```python
from build123d import *

# Parameters (mm, degrees)
SKETCH1_R           = 4
BOSS_EXTRUDE1_DEPTH = 25
SKETCH2_R           = 10
CUT_EXTRUDE1_DEPTH  = 15


with BuildPart() as part:
    # Sketch1 → Boss-Extrude1 (new body)
    with BuildSketch(Plane(origin=(0, 0, 0), x_dir=(1, 0, 0), z_dir=(0, 1, 0))):
        Polygon((-35, -10), (-30, -10), (-30, -25), (30, -25), (30, -10), (35, -10), (35, 10), (-35, 10), align=None)
        with Locations(Location((-25, 0, 0), (0, 0, 270))):
            Circle(SKETCH1_R, mode=Mode.SUBTRACT)
        with Locations(Location((25, 0, 0), (0, 0, 90))):
            Circle(SKETCH1_R, mode=Mode.SUBTRACT)
    extrude(amount=BOSS_EXTRUDE1_DEPTH)

    # Sketch2 → Cut-Extrude1 (cut)
    with BuildSketch(Plane.XY.offset(25)):
        with Locations((-12.5, 12.5)):
            Circle(SKETCH2_R)
        with Locations(Location((12.5, 12.5, 0), (0, 0, 180))):
            Circle(SKETCH2_R)
    extrude(amount=-CUT_EXTRUDE1_DEPTH, mode=Mode.SUBTRACT)


solid = part.part
```
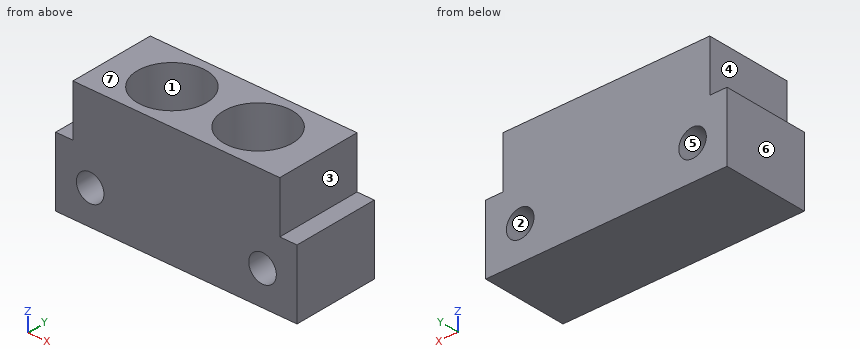
Source: CAD feature listing. Evaluate the final solid. Frame: model axes, mm. Face numbers are marked on the shaded views. A direction names the side the tool comes from. Round coordinates to 2 decimals unless told otherwise and drop trailing zeros. Loops run counter-clockwise (first coordinate to the right, second up) from the corner with the lowest first, then second, coordinate; pieces in that order, holes last. Notation, with made-up numbers: M 88.25,-24 L 135.25,-24 A8 cw 135.25,-18 Z; hole C 75,83.25 d6. An arc over 180 degrees is marked long. Put each result on its own line as item: value.
(1) Access query for the marked faces 1, 2, 3 and 4. Directions: +Z, -Z, +X, -X, +Y, -Y. A direction counts if a zero-diameter tool reaches every point of the face in a straight line with its end or side. Return the directions, or none.
Solutions:
face 1: +Z
face 2: +Y, -Y
face 3: +Z, +X, +Y, -Y
face 4: +Z, -X, +Y, -Y
(2) Ray query, line 1 (X direction, y = 16, z = 0); line 2 (X direction, y = 21, z = 18.5); line 3 (Y direction, x = 12.5, z = 15.25). Return the intervals inside material, ascending. Write a range as [from, to].
Solutions:
line 1: [-35, -29], [-21, 21], [29, 35]
line 2: [-30, -17.77], [-7.23, 7.23], [17.77, 30]
line 3: [0, 2.5], [22.5, 25]
(3) First-contact query: pin 1 (7.5 mm diameter, centred on y = 7.5, z = 18, fed in from +X); pin 2 (3 mm diameter, centred on x = -12, y = 5, fed in from +Z); pin 3 (7.5 mm diameter, centred on y = 9, z = 21, fed in from -X). Flat tips, straight axial feed; report the tip coordinate or a pass-through.
Solutions:
pin 1: x = 30
pin 2: z = 10
pin 3: x = -30
(4) Section C-C, the plane x = 12.5. Return loops of the section in (y, z), and give its area (3 significant figures).
Solutions:
outline: M 0,-10 L 25,-10 L 25,25 L 22.5,25 L 22.5,10 L 2.5,10 L 2.5,25 L 0,25 Z
area: 575 mm²
(5) Section A-A, the plane z = 0. Return loops of the section in (x, y), and give its area (3 significant figures).
Solutions:
outline: M -35,0 L -29,0 L -29,25 L -35,25 Z; M -21,0 L 21,0 L 21,25 L -21,25 Z; M 29,0 L 35,0 L 35,25 L 29,25 Z
area: 1,350 mm²
(6) Section D-D, the plane y = 11.25. Return loops of the section in (x, z).
Solutions:
outline: M -35,-10 L 35,-10 L 35,10 L 30,10 L 30,25 L 22.42,25 L 22.42,10 L 2.58,10 L 2.58,25 L -2.58,25 L -2.58,10 L -22.42,10 L -22.42,25 L -30,25 L -30,10 L -35,10 Z; hole C -25,0 d8; hole C 25,0 d8
(7) Pull-direction query (X, two-part tool) for the marked faces 5, 6 and 7; classes: released by +X, released by -X, zero draft, split by the parting line, or undercut.
Solutions:
face 5: undercut
face 6: released by -X
face 7: zero draft
(8) Section B-B, the plane x = 25. Return loops of the section in (y, z), and give its area (3 significant figures).
Solutions:
outline: M 0,-10 L 25,-10 L 25,-4 L 0,-4 Z; M 0,4 L 25,4 L 25,25 L 0,25 Z
area: 675 mm²
